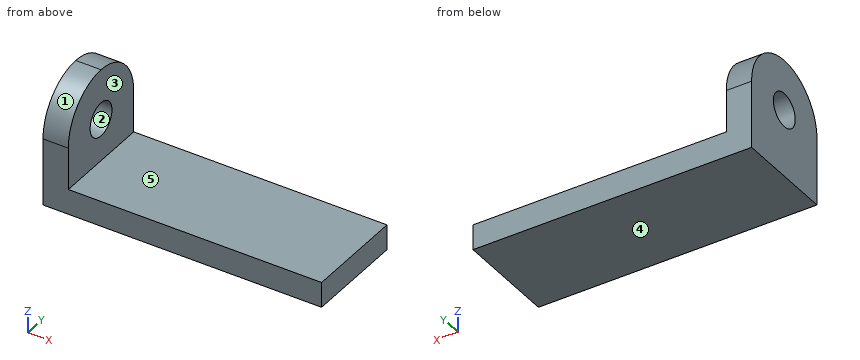
```python
from build123d import *

# Parameters (mm, degrees)
F0_W     = 167.64
F0_H     = 60.96
F1_DEPTH = 15.24
F2_W     = 15.24
F2_H     = 60.96
F3_DEPTH = 55.88
F4_R     = 30.47999
F5_R     = 10.16
F6_DEPTH = 15.24


# Not quite as in the source:
# - a fillet or chamfer is up to 0.001 mm smaller than in the source, because OpenCascade refuses the exact size


with BuildPart() as f1:
    # F0 (on Top) → F1 (new body)
    with BuildSketch(Plane.XY):
        with Locations((50.7921350074, 13.222941007)):
            Rectangle(F0_W, F0_H)
    extrude(amount=F1_DEPTH)

    # F2 (on face) → F3 (join)
    with BuildSketch(Plane.XY.offset(15.24)):
        with Locations((-25.4078649926, 13.222941007)):
            Rectangle(F2_W, F2_H)
    extrude(amount=F3_DEPTH)

    # F4 (radius 30.48 in the source; OpenCascade refuses exactly that, so slightly less here)
    f4_edges = [f1.edges().sort_by_distance(p)[0] for p in [
        (-25.407865, -17.257059, 71.12),
        (-25.407865, 43.702941, 71.12),
    ]]
    fillet(f4_edges, radius=F4_R)

    # F5 (on face) → F6 (cut)
    with BuildSketch(Plane(origin=(-33.0278649926, 0, 0), x_dir=(0, -1, 0), z_dir=(-1, 0, 0))):
        with Locations((-13.222941007, 40.64)):
            Circle(F5_R)
    extrude(amount=-F6_DEPTH, mode=Mode.SUBTRACT)


solid = f1.part
```
Work out the finished part from the listing and answer in its coordinate system (mm). Face numbers are marked on the shaded views. A direction names the side the tool comes from. Give positions to 0.01 mm unless a question says otherwise; leave off trailing zeros. Loops run counter-clockwise (first coordinate to the right, second up) from the corner with the lowest first, then second, coordinate; pieces in that order, holes last. Notation, with made-up numbers: (15, -0.5) -> (62, -0.5) arc R31 ccw to (62, 29.5) -> close; hole circle Ø7 at (50, 42.5). An arc over 180 degrees is marked (long way). Put each result on its own line as item: value. Start each with the question number.
Item 1: Find the intervals of material crossed by L1, parallel to X at y = 22.5, z = 57.5; L2, parallel to Z at x = 52, y = 4.5; L3, parallel to Y at x = -29, z = 40, in increasing order. Write a range as [from, to].
Item 2: The part is cut by section C-C (z = 65). Give the vertices of the cut face in (x, y), then the cut area to 3 significant figures.
Item 3: The mould has two halves that part along Y. Classify the marked faces 1, 2 and 3: released by +Y, released by -Y, zero draft, split by the parting line, or undercut.
Item 4: The part is cut by section A-A (x = 106). Give the vertices of the cut face in (y, z).
Item 5: Each of these flat-tipped pins is pushed along its axis until it touches: P1, Ø6, axis at x = 12, y = 33, coming from the +Z side; P2, Ø18.5, axis at y = 13.22, z = 40.64, coming from the -X side. Where does it stop, or does it pass through?
Item 6: Which of the six approach directions +Z, -Z, +X, -X, +Y, -Y give full straight-line access (tool end or side, diameter ignored) to the marked faces 4 and 5?
Item 7: The part is cut by section B-B (y = -1.5). Give the vertices of the cut face in (x, z).
Answers below:
1. L1: [-33.03, -17.79]
1. L2: [0, 15.24]
1. L3: [-17.26, 3.08], [23.36, 43.7]
2. outline: (-33.03, -5.1) -> (-17.79, -5.1) -> (-17.79, 31.54) -> (-33.03, 31.54) -> close
2. area: 558 mm2
3. face 1: released by -Y
3. face 2: undercut
3. face 3: zero draft
4. outline: (-17.26, 0) -> (43.7, 0) -> (43.7, 15.24) -> (-17.26, 15.24) -> close
5. P1: z = 15.24
5. P2: through
6. face 4: -Z, +X, -X, +Y, -Y
6. face 5: +Z, +X, +Y, -Y
7. outline: (-33.03, 0) -> (134.61, 0) -> (134.61, 15.24) -> (-17.79, 15.24) -> (-17.79, 67.33) -> (-33.03, 67.33) -> close
